Source: CAD feature listing. Evaluate the final solid. Frame: model axes, mm. Face numbers are marked on the shaded views. Coordinates: 2 decimals unless noted, no trailing zeros. Loops run counter-clockwise (first coordinate to the right, second up) from the corner with the lowest first, then second, coordinate; pieces in that order, holes last.
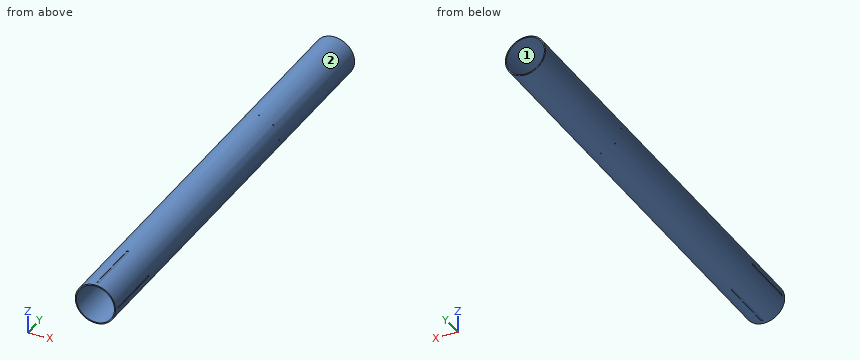
from build123d import *

# Parameters (mm, degrees)
SKETCH1_R                 = 53.721
SKETCH1_R_2               = 50.8
BODY_TUBE_EXTRUSION_DEPTH = 1206.5
BULKHEAD_HOLE_REACH       = 1214.465
BULKHEAD_HOLE_END_RADIUS  = 50.8
SKETCH2_R                 = 1.6383
CIRPATTERN1_COUNT         = 8
SKETCH3_W                 = 5.334
SKETCH3_H                 = 152.4
CUT_EXTRUDE1_DEPTH        = 1.27
CIRPATTERN2_COUNT         = 4


with BuildPart() as part:
    # Sketch1 → Body Tube Extrusion (new body)
    with BuildSketch(Plane(origin=(0, 0, 0), x_dir=(1, 0, 0), z_dir=(0, 1, 0))):
        Circle(SKETCH1_R)
        Circle(SKETCH1_R_2, mode=Mode.SUBTRACT)
    extrude(amount=BODY_TUBE_EXTRUSION_DEPTH)

    # Bulkhead Hole: up to this cylinder (the profile starts outside it)
    bulkhead_hole_end = Plane(origin=(0, 825.5, 0), z_dir=(0, -1, 0)) * Cylinder(BULKHEAD_HOLE_END_RADIUS, 2531.53, mode=Mode.PRIVATE)
    # Sketch2 → Bulkhead Hole (cut, up to the surface)
    with BuildSketch(Plane.XY.offset(53.721), mode=Mode.PRIVATE) as bulkhead_hole_sk1:
        with Locations((0, 825.5)):
            Circle(SKETCH2_R)
    bulkhead_hole_tool1 = extrude(bulkhead_hole_sk1.sketch, amount=-BULKHEAD_HOLE_REACH, mode=Mode.PRIVATE) - bulkhead_hole_end
    bulkhead_hole = bulkhead_hole_tool1.solids().sort_by_distance((0, 825.5, 53.721))[0]
    add(bulkhead_hole, mode=Mode.SUBTRACT)

    # CirPattern1: Bulkhead Hole ×8 about axis
    cirpattern1_axis = Axis((0, 1206.5, 0), (0, -1, 0))
    for i in range(1, CIRPATTERN1_COUNT):
        add(bulkhead_hole.rotate(cirpattern1_axis, i * 360 / CIRPATTERN1_COUNT), mode=Mode.SUBTRACT)

    # Sketch3 → Cut-Extrude1 (cut)
    with BuildSketch(Plane.XY.offset(53.721)):
        with Locations((0, 88.9)):
            Rectangle(SKETCH3_W, SKETCH3_H)
    cut_extrude1 = extrude(amount=-CUT_EXTRUDE1_DEPTH, mode=Mode.SUBTRACT)

    # CirPattern2: Cut-Extrude1 ×4 about axis
    cirpattern2_axis = Axis((0, 0, 0), (0, 1, 0))
    for i in range(1, CIRPATTERN2_COUNT):
        add(cut_extrude1.rotate(cirpattern2_axis, i * 360 / CIRPATTERN2_COUNT), mode=Mode.SUBTRACT)


solid = part.part
Q1. Draft query along Z for the marked faces 1 and 2. Return one class per face: +Z half, -Z half, draft (parallel to the pull), parting line (faces both ways), or undercut.
Q2. Contact query for flat-ended pins moving along their axis: pin 1 Ø4 at (y, z) = (975, 28.5) entering from +X; pin 2 Ø6 at (x, y) = (-27.5, 697.5) entering from +Z; pin 3 Ø2 at (y, z) = (485, -25.5) entering from +X. Output: stop coordinate, or through.
Q3. Section C-C, the plane y = 846.5. Return the cut outline in (x, z).
Q4. Line query: line 1 along Y through (x, z) = (0, -52.7); line 2 along Z through (x, y) = (3.5, 846.5); line 3 along X through (y, z) = (81.5, -5). Output: solid intervals per line, ascending.
Q5. Section A-A, the plane z = -24. Return the cut outline in (x, y).
Q6. Section B-B, the plane x = -16.5. Return the cut outline in (y, z), plus the area to 3 significant figures.
Derived:
1. face 1: undercut
1. face 2: parting line
2. pin 1: stops at x = 46.73
2. pin 2: stops at z = 47.81
2. pin 3: stops at x = 47.81
3. outline: circle Ø107.44 at (0, 0); hole circle Ø101.6 at (0, 0)
4. line 1: y = 0 to 12.7, 165.1 to 823.86, 827.14 to 1206.5
4. line 2: z = -53.61 to -50.68, 50.68 to 53.61
4. line 3: x = -53.49 to -50.55, 50.55 to 53.49
5. outline: (-48.06, 0) - (-44.77, 0) - (-44.77, 1206.5) - (-48.06, 1206.5) - close; (44.77, 0) - (48.06, 0) - (48.06, 1206.5) - (44.77, 1206.5) - close
6. outline: (0, -51.12) - (1206.5, -51.12) - (1206.5, -48.05) - (0, -48.05) - close; (0, 48.05) - (1206.5, 48.05) - (1206.5, 51.12) - (0, 51.12) - close
6. area: 7,430 mm2
